```python
from build123d import *

# Parameters (mm, degrees)
F0_W     = 770
F0_H     = 390
F1_DEPTH = 37
F2_W     = 37
F2_H     = 390
F2_W_2   = 16
F3_DEPTH = 692
F4_W     = 770
F4_H     = 390
F5_DEPTH = 39
F6_W     = 390
F6_H     = 12
F7_DEPTH = 704


with BuildPart() as f1:
    # F0 (on Top) → F1 (new body)
    with BuildSketch(Plane.XY):
        with Locations((385, 195)):
            Rectangle(F0_W, F0_H)
    extrude(amount=F1_DEPTH)

    # F2 (on face) → F3 (join)
    with BuildSketch(Plane.XY.offset(37)):
        with Locations((18.5, 195)):
            Rectangle(F2_W, F2_H)
        with Locations((751.5, 195)):
            Rectangle(F2_W, F2_H)
        with Locations((385, 195)):
            Rectangle(F2_W_2, F2_H)
    extrude(amount=F3_DEPTH)

    # F4 (on face) → F5 (join)
    with BuildSketch(Plane.XY.offset(729)):
        with Locations((385, 195)):
            Rectangle(F4_W, F4_H)
    extrude(amount=F5_DEPTH)

    # F6 (on face) → F7 (join)
    with BuildSketch(Plane(origin=(733, 0, 0), x_dir=(0, -1, 0), z_dir=(-1, 0, 0))):
        with Locations((-195, 383)):
            Rectangle(F6_W, F6_H)
    extrude(amount=F7_DEPTH)


solid = f1.part
```
Could you check a few things on this model? Use its own coordinates, in mm. A direction names the side the tool comes from. Coordinates: 2 decimals unless noted, no trailing zeros. Order: outer loops, then holes, each group sorted by start corner. A loop starts at its lowest first (then second) coordinate and runs counter-clockwise, first axis right, second up. Notation, with made-up numbers: M 49.25,-25.5 L 104.25,-25.5 A20 cw 104.25,-20.5 Z; hole C 89.5,-4.5 d7. An arc over 180 degrees is marked long. Use one line per item in the form item = value. Start each with the question number.
1. We'd pull the mould along Z, two halves only. Please class faces 1 (the flat face through (0, 192, 379)), 2 (the flat face through (380, 198, 0)), 3 (the flat face through (561, 198, 37)): +Z half, -Z half, draft (parallel to the pull), parting line (faces both ways), or undercut.
2. Suppose I cut it at B-B on z = 596. Write out the boundary of the cut face in (x, y), then the cut area to 3 significant figures.
3. On a 3-axis mill with a long thin cutter (end or side, diameter ignored), from which of +Z, -Z, +X, -X, +Y, -Y can I reach the whole of each face in a straight line? I mean faces 4 (the flat face through (770, 192, 379)), 5 (the flat face through (565, 198, 389)). Say none if no direction works.
4. Suppose I cut it at C-C on y = 83.5. Write out the boundary of the cut face in (x, z).
5. Please list where these lines run through material, in increasing order: line 1 (X direction, y = 290.5, z = 134.5); line 2 (Z direction, x = 330.5, y = 190.5).
6. Suppose I cut it at A-A on x = 201. Write out the boundary of the cut face in (y, z).
Geometry says:
q1.face_1 = draft
q1.face_2 = -Z half
q1.face_3 = undercut
q2.outline = M 0,0 L 37,0 L 37,390 L 0,390 Z; M 377,0 L 393,0 L 393,390 L 377,390 Z; M 733,0 L 770,0 L 770,390 L 733,390 Z
q2.area = 35,100 mm^2
q3.face_4 = +Z, -Z, +X, +Y, -Y
q3.face_5 = +Y, -Y
q4.outline = M 0,0 L 770,0 L 770,768 L 0,768 Z; hole M 37,37 L 377,37 L 377,377 L 37,377 Z; hole M 37,389 L 377,389 L 377,729 L 37,729 Z; hole M 393,37 L 733,37 L 733,377 L 393,377 Z; hole M 393,389 L 733,389 L 733,729 L 393,729 Z
q5.line_1 = 0 to 37, 377 to 393, 733 to 770
q5.line_2 = 0 to 37, 377 to 389, 729 to 768
q6.outline = M 0,0 L 390,0 L 390,37 L 0,37 Z; M 0,377 L 390,377 L 390,389 L 0,389 Z; M 0,729 L 390,729 L 390,768 L 0,768 Z
